from build123d import *

# Parameters (mm, degrees)
BOSS_EXTRUDE1_DEPTH = 10
SKETCH5_R           = 6.5
CUT_EXTRUDE1_DEPTH  = 10
SKETCH7_R           = 9.5
CUT_EXTRUDE2_DEPTH  = 6
SKETCH8_R           = 2.25
CUT_EXTRUDE3_DEPTH  = 15


with BuildPart() as part:
    # Sketch1 → Boss-Extrude1 (new body)
    with BuildSketch(Plane.XY):
        Polygon((-42.953588015, -13.19658427), (8.046411985, -13.19658427), (8.046411985, -3.19658427), (-1.953588015, -3.19658427), (-1.953588015, 16.80341573), (-32.953588015, 16.80341573), (-32.953588015, -3.19658427), (-42.953588015, -3.19658427), align=None)
    extrude(amount=BOSS_EXTRUDE1_DEPTH)

    # Sketch5 → Cut-Extrude1 (cut)
    with BuildSketch(Plane(origin=(0, 0, 0), x_dir=(-1, 0, 0), z_dir=(0, 0, -1))):
        with Locations((17.453588015, 1.30341573)):
            Circle(SKETCH5_R)
    extrude(amount=-CUT_EXTRUDE1_DEPTH, mode=Mode.SUBTRACT)

    # Sketch7 → Cut-Extrude2 (cut)
    with BuildSketch(Plane(origin=(0, 0, 0), x_dir=(-1, 0, 0), z_dir=(0, 0, -1))):
        with Locations((17.453588015, 1.30341573)):
            Circle(SKETCH7_R)
    extrude(amount=-CUT_EXTRUDE2_DEPTH, mode=Mode.SUBTRACT)

    # Sketch8 → Cut-Extrude3 (cut)
    with BuildSketch(Plane(origin=(0, -3.19658427, 0), x_dir=(1, 0, 0), z_dir=(0, 1, 0))):
        with Locations(Location((3.046411985, -5, 0), (0, 0, 180))):
            Circle(SKETCH8_R)
        with Locations(Location((-37.953588015, -5, 0), (0, 0, 180))):
            Circle(SKETCH8_R)
    extrude(amount=-CUT_EXTRUDE3_DEPTH, mode=Mode.SUBTRACT)


solid = part.part
The model under review builds one solid part; all positions refer to its coordinate system, in mm. A direction names the side the tool comes from. Round coordinates to 2 decimals unless told otherwise and drop trailing zeros. Loops run counter-clockwise (first coordinate to the right, second up) from the corner with the lowest first, then second, coordinate; pieces in that order, holes last. Notation, with made-up numbers: (-31, 68) -> (21, 68) arc R11 cw to (21, 78) -> close; hole circle Ø8 at (64.25, 89.25). An arc over 180 degrees is marked (long way). Return JSON: item names as keys, results as strings.
(1) For faces 4 (the flat face through (-35.7, -3.197, 3.8)), 5 (the flat face through (4.2, -3.197, 2.7)), 6 (the cylindrical face through (-22.561, 9.314, 2.958)), list the 3-axis set-ups (+Z, -Z, +X, -X, +Y, -Y) from which the entire face can be reached by the end or side of a thin tool; tool diameter is ignored.
Solved:
{"face 4": "+Z, -Z, -X, +Y", "face 5": "+Z, -Z, +X, +Y", "face 6": "-Z"}
(2) Add section D-D on y = -7.5. Write out the cut boundary in (x, z).
Solved:
{"outline": "(-42.95, 0) -> (-21.02, 0) -> (-21.02, 6) -> (-13.88, 6) -> (-13.88, 0) -> (8.05, 0) -> (8.05, 10) -> (-42.95, 10) -> close; hole circle Ø4.5 at (-37.95, 5); hole circle Ø4.5 at (3.05, 5)"}
(3) Add section B-B on x = -13. Write out the cut boundary in (y, z).
Solved:
{"outline": "(-13.2, 0) -> (-7.09, 0) -> (-7.09, 6) -> (-3.43, 6) -> (-3.43, 10) -> (-13.2, 10) -> close; (6.04, 6) -> (9.69, 6) -> (9.69, 0) -> (16.8, 0) -> (16.8, 10) -> (6.04, 10) -> close"}
(4) For line 1 (Y direction, x = -0.5, z = 2.75); line 2 (X direction, y = 11, z = 8.25); line 3 (Y direction, x = -16, z = 7), list the stretches that pass through material, from the lowest coordinate up.
Solved:
{"line 1": "-13.2 to -3.2", "line 2": "-32.95 to -1.95", "line 3": "-13.2 to -5.03, 7.64 to 16.8"}
(5) The part is to be moulded in two halves that separate along X. For faces 1 (the flat face through (-32.954, 7, 5)), 2 (the flat face through (-24, -1, 6)), 3 (the flat face through (-23, -8, 0)), say which applies: released by +X, released by -X, zero draft, split by the parting line, or undercut.
Solved:
{"face 1": "released by -X", "face 2": "undercut", "face 3": "zero draft"}
(6) For pin 1 (3 mm diameter, centred on y = 6, z = 4, fed in from +X); pin 2 (3 mm diameter, centred on x = 1, z = 5.5, fed in from +Y); pin 3 (5 mm diameter, centred on y = 5, z = 3.5, fed in from -X), all flat-tipped, find the tip position at first contact; note any pin that passes through.
Solved:
{"pin 1": "x = -1.95", "pin 2": "y = -3.2", "pin 3": "x = -32.95"}
(7) Add section C-C on y = -1.5. Write out the cut boundary in (x, z).
Solved:
{"outline": "(-32.95, 0) -> (-26.53, 0) -> (-26.53, 6) -> (-23.32, 6) -> (-23.32, 10) -> (-32.95, 10) -> close; (-11.59, 6) -> (-8.38, 6) -> (-8.38, 0) -> (-1.95, 0) -> (-1.95, 10) -> (-11.59, 10) -> close"}
(8) Add section A-A on z = 4.5. Write out the cut boundary in (x, y), plus the area to 3 significant figures.
Solved:
{"outline": "(-42.95, -13.2) -> (-40.15, -13.2) -> (-40.15, -3.2) -> (-42.95, -3.2) -> close; (-35.76, -13.2) -> (0.85, -13.2) -> (0.85, -3.2) -> (-1.95, -3.2) -> (-1.95, 16.8) -> (-32.95, 16.8) -> (-32.95, -3.2) -> (-35.76, -3.2) -> close; (5.24, -13.2) -> (8.05, -13.2) -> (8.05, -3.2) -> (5.24, -3.2) -> close; hole circle Ø19 at (-17.45, 1.3)", "area": "759 mm2"}
